Could you check a few things on this model? Use its own coordinates, in mm. Round coordinates to 2 decimals unless told otherwise and drop trailing zeros. Write each loop counter-clockwise with the first axis right and the second up, starting at its lowest first coordinate (ties: lowest second). Pieces come first, ordered by that corner, then holes. Notation, with made-up numbers: (-16, 74) - (29, 74) arc R29 ccw to (29, 102) - close; hole circle Ø3 at (72.25, 0.5). An arc over 180 degrees is marked (long way). Put each result on its own line as item: value.
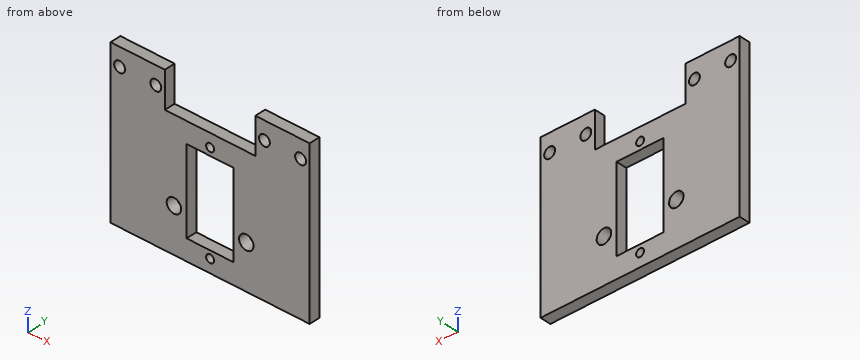
from build123d import *

# Parameters (mm, degrees)
SKETCH1_R           = 1.5
SKETCH1_R_2         = 1.1
SKETCH1_W           = 13
SKETCH1_H           = 23.5
BOSS_EXTRUDE1_DEPTH = 3
SKETCH2_R           = 2
CUT_EXTRUDE1_DEPTH  = 72.126647608


with BuildPart() as part:
    # Sketch1 → Boss-Extrude1 (new body)
    with BuildSketch(Plane(origin=(0, 0, 0), x_dir=(1, 0, 0), z_dir=(0, 1, 0))):
        Polygon((0, 0), (15, 0), (15, 10), (40, 10), (40, 0), (55, 0), (55, 45), (0, 45), align=None)
        with Locations(Location((42.5, 5, 0), (0, 0, 270))):
            Circle(SKETCH1_R, mode=Mode.SUBTRACT)
        with Locations(Location((52.5, 5, 0), (0, 0, 270))):
            Circle(SKETCH1_R, mode=Mode.SUBTRACT)
        with Locations(Location((12.5, 5, 0), (0, 0, 270))):
            Circle(SKETCH1_R, mode=Mode.SUBTRACT)
        with Locations(Location((2.5, 5, 0), (0, 0, 270))):
            Circle(SKETCH1_R, mode=Mode.SUBTRACT)
        with Locations(Location((27.5, 41.35, 0), (0, 0, 270))):
            Circle(SKETCH1_R_2, mode=Mode.SUBTRACT)
        with Locations(Location((27.5, 13.65, 0), (0, 0, 90))):
            Circle(SKETCH1_R_2, mode=Mode.SUBTRACT)
        with Locations((27.5, 27.5)):
            Rectangle(SKETCH1_W, SKETCH1_H, mode=Mode.SUBTRACT)
    extrude(amount=BOSS_EXTRUDE1_DEPTH)

    # Sketch2 → Cut-Extrude1 (cut, through all)
    with BuildSketch(Plane(origin=(0, 3, 0), x_dir=(1, 0, 0), z_dir=(0, 1, 0))):
        with Locations(Location((17.5, 32.699969783, 0), (0, 0, 270))):
            Circle(SKETCH2_R)
        with Locations(Location((37.5, 32.699969783, 0), (0, 0, 90))):
            Circle(SKETCH2_R)
    extrude(amount=-CUT_EXTRUDE1_DEPTH, mode=Mode.SUBTRACT)


solid = part.part
(1) Please list where these lines run through material, in increasing order: probe 1 along X at (y, z) = (2.3, -5); probe 2 along Z at (x, y) = (21.5, 1.65); probe 3 along X at (y, z) = (2.35, -38). Write a range as from..to.
Values found:
probe 1: x = 0..1, 4..11, 14..15, 40..41, 44..51, 54..55
probe 2: z = -45..-39.25, -15.75..-10
probe 3: x = 0..21, 34..55
(2) Imagine slicing it at B-B, the plane x = 12.5. List the corners of the cut face in (y, z) for me.
Values found:
outline: (0, -45) - (3, -45) - (3, -6.5) - (0, -6.5) - close; (0, -3.5) - (3, -3.5) - (3, 0) - (0, 0) - close
(3) Imagine slicing it at A-A, the plane z = -13.65. List the corners of the cut face in (x, y) for me.
Values found:
outline: (0, 0) - (26.4, 0) - (26.4, 3) - (0, 3) - close; (28.6, 0) - (55, 0) - (55, 3) - (28.6, 3) - close
(4) I'm going to push flat-ended pins straight in: pin 1 (1.5 mm diameter, centred on x = 33, y = 2, fed in from +Z); pin 2 (2.5 mm diameter, centred on x = 2.5, z = -5, fed in from +Y). Where does each tip first touch, or does it pass through?
Values found:
pin 1: stops at z = -10
pin 2: passes through
(5) Imagine slicing it at D-D, the plane y = 2.2. Give the number of separate pieces and of enclosed holes in the cut face, then the cut area to 3 significant figures.
Values found:
separate pieces: 1
enclosed holes: 9
area: 1,860 mm^2
(6) Imagine slicing it at C-C, the plane x = 27.5. List the corners of the cut face in (y, z) for me, then the cut area to 3 significant figures.
Values found:
outline: (0, -45) - (3, -45) - (3, -42.45) - (0, -42.45) - close; (0, -40.25) - (3, -40.25) - (3, -39.25) - (0, -39.25) - close; (0, -15.75) - (3, -15.75) - (3, -14.75) - (0, -14.75) - close; (0, -12.55) - (3, -12.55) - (3, -10) - (0, -10) - close
area: 21.3 mm^2
